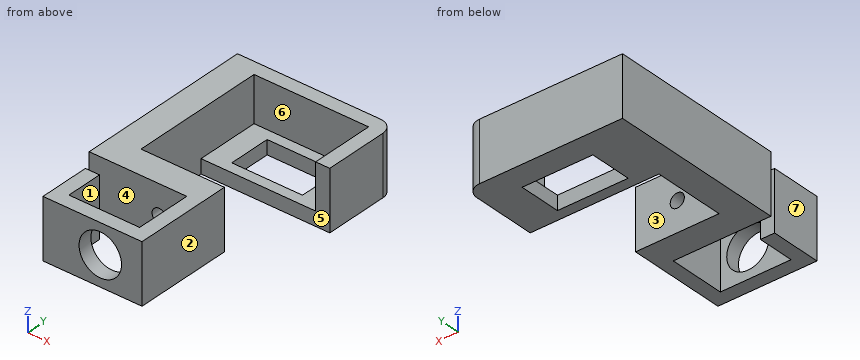
from build123d import *

# Parameters (mm, degrees)
SKETCH_W        = 25
SKETCH_H        = 15
PAD_DEPTH       = 5
PAD001_DEPTH    = 16
SKETCH002_R     = 2.5
SKETCH002_W     = 16
SKETCH002_H     = 21
POCKET_DEPTH    = 15
SKETCH003_W     = 5
SKETCH003_H     = 21
PAD002_DEPTH    = 25
SKETCH004_W     = 5
SKETCH004_H     = 21
PAD003_DEPTH    = 30
SKETCH005_W     = 5
SKETCH005_H     = 21
PAD004_DEPTH    = 13
SKETCH006_R     = 7.5
POCKET001_DEPTH = 10


with BuildPart() as part:
    # Sketch → Pad (new body)
    with BuildSketch(Plane.XY):
        with BuildLine():
            Line((0, -35.5), (0, 27.5))
            Line((0, 27.5), (50.5, 27.5))
            ThreePointArc((55.5, 22.5), (54.035534, 26.035534), (50.5, 27.5))
            Line((55.5, 22.5), (55.5, 0))
            Line((55.5, 0), (10, 0))
            Line((10, 0), (10, -25.5))
            Line((10, -25.5), (55.5, -25.5))
            Line((55.5, -25.5), (55.5, -35.5))
            Line((55.5, -35.5), (0, -35.5))
        make_face()
        with Locations((30.25, 11.25)):
            Rectangle(SKETCH_W, SKETCH_H, mode=Mode.SUBTRACT)
    extrude(amount=PAD_DEPTH)

    # Sketch001 (on Face15 of Pad) → Pad001 (join)
    with BuildSketch(Plane.XY.offset(5)):
        with BuildLine():
            Line((55.5, 22.5), (55.5, 0))
            Line((55.5, 0), (50.5, 0))
            Line((50.5, 0), (50.5, 22.5))
            Line((50.5, 22.5), (10, 22.5))
            Line((10, 22.5), (10, -25.5))
            Line((55.5, -25.5), (10, -25.5))
            Line((55.5, -35.5), (55.5, -25.5))
            Line((0, -35.5), (55.5, -35.5))
            Line((0, 27.5), (0, -35.5))
            Line((50.5, 27.5), (0, 27.5))
            ThreePointArc((55.5, 22.5), (54.035534, 26.035534), (50.5, 27.5))
        make_face()
    extrude(amount=PAD001_DEPTH)

    # Sketch002 (on Face26 of Pad001) → Pocket (cut)
    with BuildSketch(Plane.XZ.offset(35.5)):
        with Locations((24.75, 10.5)):
            Circle(SKETCH002_R)
        with Locations((47.5, 10.5)):
            Rectangle(SKETCH002_W, SKETCH002_H)
    extrude(amount=-POCKET_DEPTH, mode=Mode.SUBTRACT)

    # Sketch003 (on Face25 of Pocket) → Pad002 (join)
    with BuildSketch(Plane.XZ.offset(35.5)):
        with Locations((37, 10.5)):
            Rectangle(SKETCH003_W, SKETCH003_H)
    extrude(amount=PAD002_DEPTH)

    # Sketch004 (on Face27 of Pad002) → Pad003 (join)
    with BuildSketch(Plane(origin=(34.5, 0, 0), x_dir=(0, -1, 0), z_dir=(-1, 0, 0))):
        with Locations((58, 10.5)):
            Rectangle(SKETCH004_W, SKETCH004_H)
    extrude(amount=PAD003_DEPTH)

    # Sketch005 (on Face34 of Pad003) → Pad004 (join)
    with BuildSketch(Plane(origin=(0, -55.5, 0), x_dir=(-1, 0, 0), z_dir=(0, 1, 0))):
        with Locations((-7, 10.5)):
            Rectangle(SKETCH005_W, SKETCH005_H)
    extrude(amount=PAD004_DEPTH)

    # Sketch006 (on Face36 of Pad004) → Pocket001 (cut)
    with BuildSketch(Plane.XZ.offset(60.5)):
        with Locations((24.75, 10.5)):
            Circle(SKETCH006_R)
    extrude(amount=-POCKET001_DEPTH, mode=Mode.SUBTRACT)


solid = part.part
The listing builds one solid part. Answer for the finished solid, in the listing's coordinates (mm). Face numbers are marked on the shaded views. A direction names the side the tool comes from. Coordinates: 2 decimals unless noted, no trailing zeros. Order: outer loops, then holes, each group sorted by start corner. A loop starts at its lowest first (then second) coordinate and runs counter-clockwise, first axis right, second up.
Q1. A cutting plane is placed at B-B, the plane x = 24.75. Write down the section's boundary in (y, z).
Q2. A cutting plane is placed at C-C, the plane z = 14.75. Write down the section's boundary in (x, y), and give its area (3 significant figures).
Q3. A cutting plane is placed at A-A, the plane z = 10.5. Write down the section's boundary in (x, y), and give its area (3 significant figures).
Q4. For a pull along X with two mould halves and no side action, classify the marked faces 5, 6 and 7 as pulls with the +X half, pulls with the -X half, needs draft (parallel to the pull), parting line crosses it, or undercut.
Q5. Which of the six approach directions +Z, -Z, +X, -X, +Y, -Y give full straight-line access (tool end or side, diameter ignored) to the marked faces 1, 2, 3 and 4?
Q6. Given P1, Ø10, axis at x = 46, z = 12, coming from the -Y side; P2, Ø6, axis at y = -49.5, z = 10, coming from the -X side; P3, Ø10.5, axis at y = -45.5, z = 15.5, coming from the +X side, each flat-ended and moving along its own axis, determine where each tip first touches the part or whether it passes through.
Q7. Consider line 1 (Y direction, x = 14, z = 4.5); line 2 (Y direction, x = 17.5, z = 13.25); line 3 (X direction, y = 14, z = 15.75). Determine where each line is inside the solid, lowest interval first.
Q8. A cutting plane is placed at D-D, the plane y = -32.5. Write down the section's boundary in (x, z).
Answers follow:
1. outline: (-60.5, 0) - (-55.5, 0) - (-55.5, 3) - (-60.5, 3) - close; (-60.5, 18) - (-55.5, 18) - (-55.5, 21) - (-60.5, 21) - close; (-35.5, 0) - (-25.5, 0) - (-25.5, 8) - (-35.5, 8) - close; (-35.5, 13) - (-25.5, 13) - (-25.5, 21) - (-35.5, 21) - close; (0, 0) - (3.75, 0) - (3.75, 5) - (0, 5) - close; (18.75, 0) - (27.5, 0) - (27.5, 21) - (22.5, 21) - (22.5, 5) - (18.75, 5) - close
2. outline: (0, -35.5) - (34.5, -35.5) - (34.5, -55.5) - (30.93, -55.5) - (30.93, -60.5) - (39.5, -60.5) - (39.5, -25.5) - (10, -25.5) - (10, 22.5) - (50.5, 22.5) - (50.5, 0) - (55.5, 0) - (55.5, 22.5) arc R5 ccw to (50.5, 27.5) - (0, 27.5) - close; (4.5, -60.5) - (18.57, -60.5) - (18.57, -55.5) - (9.5, -55.5) - (9.5, -42.5) - (4.5, -42.5) - close
2. area: 1,540 mm2
3. outline: (0, -35.5) - (22.25, -35.5) - (22.25, -25.5) - (10, -25.5) - (10, 22.5) - (50.5, 22.5) - (50.5, 0) - (55.5, 0) - (55.5, 22.5) arc R5 ccw to (50.5, 27.5) - (0, 27.5) - close; (4.5, -60.5) - (17.25, -60.5) - (17.25, -55.5) - (9.5, -55.5) - (9.5, -42.5) - (4.5, -42.5) - close; (27.25, -35.5) - (34.5, -35.5) - (34.5, -55.5) - (32.25, -55.5) - (32.25, -60.5) - (39.5, -60.5) - (39.5, -25.5) - (27.25, -25.5) - close
3. area: 1,470 mm2
4. face 5: needs draft
4. face 6: undercut
4. face 7: pulls with the -X half
5. face 1: +Z, -Z
5. face 2: +Z, -Z, +X, -Y
5. face 3: +Z, -Z, +X
5. face 4: +Z, -Z, -X
6. P1: stops at y = 0
6. P2: stops at x = 4.5
6. P3: stops at x = 39.5
7. line 1: y = -60.5 to -55.5, -35.5 to -25.5, 0 to 27.5
7. line 2: y = -60.5 to -55.5, -35.5 to -25.5, 22.5 to 27.5
7. line 3: x = 0 to 10, 50.5 to 55.5
8. outline: (0, 0) - (39.5, 0) - (39.5, 21) - (0, 21) - close; hole circle Ø5 at (24.75, 10.5)
